```python
from build123d import *

# Parameters (mm, degrees)
SKETCH2_R               = 12.5
BOSS_EXTRUDE2_DEPTH     = 25
SKETCH3_R               = 3.4
CUT_EXTRUDE1_DEPTH      = 30
SKETCH4_R               = 1.25
CUT_EXTRUDE2_DEPTH      = 13.5
CUT_EXTRUDE2_DEPTH_BACK = 2.5
BOSS_EXTRUDE3_DEPTH     = 10
FILLET2_R               = 3


with BuildPart() as part:
    # Sketch2 → Boss-Extrude2 (new body)
    with BuildSketch(Plane(origin=(0, 0, 0), x_dir=(1, 0, 0), z_dir=(0, 1, 0))):
        Circle(SKETCH2_R)
    extrude(amount=BOSS_EXTRUDE2_DEPTH)

    # Sketch3 → Cut-Extrude1 (cut)
    with BuildSketch(Plane(origin=(0, 25, 0), x_dir=(1, 0, 0), z_dir=(0, 1, 0))):
        Circle(SKETCH3_R)
    extrude(amount=-CUT_EXTRUDE1_DEPTH, mode=Mode.SUBTRACT)

    # Sketch4 → Cut-Extrude2 (cut, two sides)
    with BuildSketch(Plane.XY) as cut_extrude2_sk:
        with Locations((0, 15)):
            Circle(SKETCH4_R)
    extrude(amount=CUT_EXTRUDE2_DEPTH, mode=Mode.SUBTRACT)
    extrude(cut_extrude2_sk.sketch, amount=-CUT_EXTRUDE2_DEPTH_BACK, mode=Mode.SUBTRACT)

    # Sketch5 → Boss-Extrude3 (add)
    with BuildSketch(Plane.XZ):
        Polygon((7.248737342, -17.5), (17.5, -7.248737342), (17.5, 7.248737342), (7.248737342, 17.5), (-7.248737342, 17.5), (-17.5, 7.248737342), (-17.5, -7.248737342), (-7.248737342, -17.5), align=None)
    extrude(amount=-BOSS_EXTRUDE3_DEPTH)

    # Fillet2
    fillet2_edges = [part.edges().sort_by_distance(p)[0] for p in [
        (-12.5, 10, 0),
    ]]
    fillet(fillet2_edges, radius=FILLET2_R)


solid = part.part
```
The listing builds one solid part. Answer for the finished solid, in the listing's coordinates (mm). A direction names the side the tool comes from. Give positions to 0.01 mm unless a question says otherwise; leave off trailing zeros. Order: outer loops, then holes, each group sorted by start corner. A loop starts at its lowest first (then second) coordinate and runs counter-clockwise, first axis right, second up. Notation, with made-up numbers: (-10, -28.75) -> (34, -28.75) arc R28 ccw to (34, 7.25) -> close; hole circle Ø2 at (-18.5, 24.25). An arc over 180 degrees is marked (long way). Answer as CSV lines item,"result". Start each with the question number.
Q1. A cutting plane is placed at C-C (y = 18.5). Determine the outline of the cut face in (x, z), then the cut area to 3 significant figures.
Q2. Given pin 1 (6 mm diameter, centred on x = 0, z = 0, fed in from +Y); pin 2 (1.5 mm diameter, centred on x = -4, y = 22.5, fed in from +Z); pin 3 (1 mm diameter, centred on x = -7.5, y = 15.5, fed in from +Z); pin 4 (3 mm diameter, centred on x = 13.5, z = -8, fed in from -Y), each flat-ended and moving along its own axis, determine where each tip first touches the part or whether it passes through.
Q3. Find the intervals of material crossed by L1, parallel to Y at x = 0, z = 6; L2, parallel to Z at x = 0, y = 18, in increasing order.
Q4. A cutting plane is placed at D-D (y = 15). Determine the outline of the cut face in (x, z), then the cut area to 3 significant figures.
Q5. A cutting plane is placed at B-B (z = 0). Determine the outline of the cut face in (x, y), then the cut area to 3 significant figures.
Q6. Which of the six approach directions +Z, -Z, +X, -X, +Y, -Y give full straight-line access (tool end or side, diameter ignored) to faces 1 (the cylindrical face through (0.672, 16.054, 7.766)), 2 (the flat face through (2.5, 10, -15.5)), 3 (the flat face through (-12.45, 4.93, -12.3))?
Q7. Determine the mould class of faces 4 (the flat face through (12.3, 4.93, -12.45)), 5 (the cylindrical face through (1.828, 17.605, -2.867)), 6 (the flat face through (-17.5, 5, 0)), 7 (the flat face through (0, 10, 0)) for opening direction X: pulls with the +X half, pulls with the -X half, needs draft (parallel to the pull), parting line crosses it, or undercut.
Q8. A cutting plane is placed at A-A (x = 0). Determine the outline of the cut face in (y, z).
Results found:
1,outline,"circle Ø25 at (0, 0); hole circle Ø6.8 at (0, 0)"
1,area,"455 mm2"
2,pin 1,"y = 10"
2,pin 2,"z = 12.07"
2,pin 3,"z = 10.36"
2,pin 4,"y = 0"
3,L1,"0 to 13.75, 16.25 to 25"
3,L2,"-12.5 to -3.4, 3.4 to 12.5"
4,outline,"(-1.25, 3.16) -> (-1.25, 12.44) arc R12.5 ccw (long way) to (1.25, 12.44) -> (1.25, 3.16) arc R3.4 cw (long way) to start"
4,area,"432 mm2"
5,outline,"(-17.5, 0) -> (17.5, 0) -> (17.5, 10) -> (15.5, 10) arc R3 cw to (12.5, 13) -> (12.5, 25) -> (3.4, 25) -> (3.4, 10) -> (-3.4, 10) -> (-3.4, 25) -> (-12.5, 25) -> (-12.5, 13) arc R3 cw to (-15.5, 10) -> (-17.5, 10) -> close"
5,area,"627 mm2"
6,face 1,"+Z"
6,face 2,"+Y"
6,face 3,"-Z, -X, +Y, -Y"
7,face 4,"pulls with the +X half"
7,face 5,"undercut"
7,face 6,"pulls with the -X half"
7,face 7,"undercut"
8,outline,"(0, -17.5) -> (10, -17.5) -> (10, -15.5) arc R3 cw to (13, -12.5) -> (25, -12.5) -> (25, -3.4) -> (10, -3.4) -> (10, 3.4) -> (13.75, 3.4) -> (13.75, 12.5) -> (13, 12.5) arc R3 cw to (10, 15.5) -> (10, 17.5) -> (0, 17.5) -> close; (16.25, 3.4) -> (25, 3.4) -> (25, 12.5) -> (16.25, 12.5) -> close"
